from build123d import *

# Parameters (mm, degrees)
SKETCH1_W           = 106
SKETCH1_H           = 142
BOSS_EXTRUDE1_DEPTH = 5
SKETCH2_W           = 106
SKETCH2_H           = 8
BOSS_EXTRUDE2_DEPTH = 33
SKETCH3_W           = 106
SKETCH3_H           = 8
BOSS_EXTRUDE3_DEPTH = 33
SKETCH4_W           = 8
SKETCH4_H           = 126
BOSS_EXTRUDE4_DEPTH = 33
SKETCH5_W           = 90
SKETCH5_H           = 15
BOSS_EXTRUDE5_DEPTH = 5
SKETCH6_W           = 34.6
SKETCH6_H           = 20.1
CUT_EXTRUDE1_DEPTH  = 10
FILLET1_R           = 3
FILLET2_R           = 5
SKETCH8_W           = 25
SKETCH8_H           = 5
CUT_EXTRUDE2_DEPTH  = 10
FILLET3_R           = 5


with BuildPart() as part:
    # Sketch1 → Boss-Extrude1 (new body)
    with BuildSketch(Plane(origin=(0, 0, 0), x_dir=(1, 0, 0), z_dir=(0, 1, 0))):
        Rectangle(SKETCH1_W, SKETCH1_H)
    extrude(amount=BOSS_EXTRUDE1_DEPTH)

    # Sketch2 → Boss-Extrude2 (add)
    with BuildSketch(Plane(origin=(0, 5, 0), x_dir=(1, 0, 0), z_dir=(0, 1, 0))):
        with Locations((0, -67)):
            Rectangle(SKETCH2_W, SKETCH2_H)
    extrude(amount=BOSS_EXTRUDE2_DEPTH)

    # Sketch3 → Boss-Extrude3 (add)
    with BuildSketch(Plane(origin=(0, 5, 0), x_dir=(1, 0, 0), z_dir=(0, 1, 0))):
        with Locations((0, 67)):
            Rectangle(SKETCH3_W, SKETCH3_H)
    extrude(amount=BOSS_EXTRUDE3_DEPTH)

    # Sketch4 → Boss-Extrude4 (add)
    with BuildSketch(Plane(origin=(0, 5, 0), x_dir=(1, 0, 0), z_dir=(0, 1, 0))):
        with Locations((-49, 0)):
            Rectangle(SKETCH4_W, SKETCH4_H)
        with Locations((49, 0)):
            Rectangle(SKETCH4_W, SKETCH4_H)
    extrude(amount=BOSS_EXTRUDE4_DEPTH)

    # Sketch5 → Boss-Extrude5 (add)
    with BuildSketch(Plane(origin=(0, 5, 0), x_dir=(1, 0, 0), z_dir=(0, 1, 0))):
        with Locations((0, -55.5)):
            Rectangle(SKETCH5_W, SKETCH5_H)
    extrude(amount=BOSS_EXTRUDE5_DEPTH)

    # Sketch6 → Cut-Extrude1 (cut)
    with BuildSketch(Plane.XY.offset(71)):
        with Locations((0, 22)):
            Rectangle(SKETCH6_W, SKETCH6_H)
    extrude(amount=-CUT_EXTRUDE1_DEPTH, mode=Mode.SUBTRACT)

    # Fillet1
    fillet1_edges = [part.edges().sort_by_distance(p)[0] for p in [
        (17.3, 32.05, 67),
        (17.3, 11.95, 67),
        (-17.3, 11.95, 67),
        (-17.3, 32.05, 67),
    ]]
    fillet(fillet1_edges, radius=FILLET1_R)

    # Fillet2
    fillet2_edges = [part.edges().sort_by_distance(p)[0] for p in [
        (53, 19, 71),
        (-53, 19, 71),
        (-53, 19, -71),
        (53, 19, -71),
    ]]
    fillet(fillet2_edges, radius=FILLET2_R)

    # Sketch8 → Cut-Extrude2 (cut)
    with BuildSketch(Plane(origin=(53, 0, 0), x_dir=(0, 0, -1), z_dir=(1, 0, 0))):
        with Locations((0.163227162, 35.5)):
            Rectangle(SKETCH8_W, SKETCH8_H)
    extrude(amount=-CUT_EXTRUDE2_DEPTH, mode=Mode.SUBTRACT)

    # Fillet3
    fillet3_edges = [part.edges().sort_by_distance(p)[0] for p in [
        (49, 33, 12.336772838),
        (49, 33, -12.663227162),
    ]]
    fillet(fillet3_edges, radius=FILLET3_R - 0.0001)  # a hair under: the kernel refuses the full size


solid = part.part
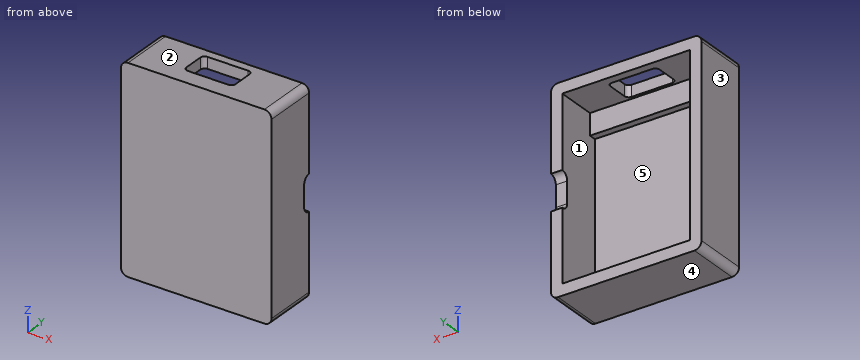
Build history of the part. All positions in model axes, mm. Face numbers are marked on the shaded views. A direction names the side the tool comes from. Coordinates: 2 decimals unless noted, no trailing zeros. Order: outer loops, then holes, each group sorted by start corner. A loop starts at its lowest first (then second) coordinate and runs counter-clockwise, first axis right, second up. Notation, with made-up numbers: (64, 20.5) -> (89, 20.5) arc R32 cw to (89, 54.5) -> close; hole circle Ø7 at (71.5, -15). An arc over 180 degrees is marked (long way). One line per item, written item: value.
(1) Slice it at A-A, the plane x = -9. List the corners of the cut face in (y, z), plus the area to 3 significant figures.
Checked values:
outline: (0, -71) -> (38, -71) -> (38, -63) -> (5, -63) -> (5, 48) -> (10, 48) -> (10, 63) -> (11.95, 63) -> (11.95, 71) -> (0, 71) -> close; (32.05, 63) -> (38, 63) -> (38, 71) -> (32.05, 71) -> close
area: 1,150 mm2
(2) Tool access for the marked faces 1 and 2: list every direction of +Z, -Z, +X, -X, +Y, -Y with a clear straight run to the whole face (end or side of a thin tool).
Checked values:
face 1: +Y
face 2: +Z, +X, -X, +Y, -Y
(3) Probe line 1 (X direction, y = 23, z = 33); line 2 (Z direction, x = -3, y = 11); line 3 (Y direction, x = 27.5, z = 50.5). List the from-to ranges inside material, lowest first. Write a range as [from, to].
Checked values:
line 1: [-53, -45], [45, 53]
line 2: [-71, -63], [63, 71]
line 3: [0, 10]
(4) Mould opens along X. For the marked faces 3, 4 and 5 say: pulls with the +X half, pulls with the -X half, needs draft (parallel to the pull), parting line crosses it, or undercut.
Checked values:
face 3: pulls with the -X half
face 4: needs draft
face 5: undercut
(5) Slice it at B-B, the plane y = 25.5. List the corners of the cut face in (x, z).
Checked values:
outline: (-53, -66) arc R5 ccw to (-48, -71) -> (48, -71) arc R5 ccw to (53, -66) -> (53, 66) arc R5 ccw to (48, 71) -> (17.3, 71) -> (17.3, 63) -> (45, 63) -> (45, -63) -> (-45, -63) -> (-45, 63) -> (-17.3, 63) -> (-17.3, 71) -> (-48, 71) arc R5 ccw to (-53, 66) -> close
(6) Slice it at C-C, the plane z = -54.5. List the corners of the cut face in (x, y), plus the area to 3 significant figures.
Checked values:
outline: (-53, 0) -> (53, 0) -> (53, 38) -> (45, 38) -> (45, 5) -> (-45, 5) -> (-45, 38) -> (-53, 38) -> close
area: 1,060 mm2
(7) Drop flat-ended pins along their axis: pin 1 Ø4 at (x, z) = (49, -1) entering from +Y; pin 2 Ø7.5 at (x, z) = (14, 52.5) entering from +Y; pin 3 Ø6 at (x, z) = (-36.5, 0) entering from +Y. Give the stop position or say it passes through.
Checked values:
pin 1: y = 33
pin 2: y = 10
pin 3: y = 5
(8) Slice it at D-D, the plane x = -32. List the corners of the cut face in (y, z).
Checked values:
outline: (0, -71) -> (38, -71) -> (38, -63) -> (5, -63) -> (5, 48) -> (10, 48) -> (10, 63) -> (38, 63) -> (38, 71) -> (0, 71) -> close
